Autodesk Inventor part; units mm, degrees
ref_plane "YZ Plane" through (0, 0, 0) normal (1, 0, 0) x (0, 1, 0)
ref_plane "XZ Plane" through (0, 0, 0) normal (0, 1, 0) x (-1, 0, 0)
ref_plane "XY Plane" through (0, 0, 0) normal (0, 0, 1) x (1, 0, 0)
sketch "Sketch1" plane through (0, 0, 0) normal (0, 0, 1) x (1, 0, 0)
  circle A0 centre (0, 0) radius 75
  line L0 (-90.1494, 78.9771) -> (78.0254, 78.9771) construction
  line L1 (78.0254, 78.9771) -> (78.0254, -87.6961) construction
  line L2 (78.0254, -87.6961) -> (-90.1494, -87.6961) construction
  line L3 (-90.1494, -87.6961) -> (-90.1494, 78.9771) construction
  line L4 (-5, 62.2697) -> (-5, 20.6534)
  line L5 (5, 20.6534) -> (5, 59.1608)
  line L6 (15.3864, 14.6568) -> (53.6249, 36.7338)
  line L7 (58.6249, 28.0736) -> (20.3864, 5.9966)
  line L8 (20.3864, -5.9966) -> (58.6249, -28.0736)
  line L9 (15.3864, -14.6568) -> (53.6249, -36.7338)
  line L10 (5, -20.6534) -> (5, -64.8074)
  line L11 (-5, -64.8074) -> (-5, -20.6534)
  line L12 (-15.3864, -14.6568) -> (-53.6249, -36.7338)
  line L13 (-58.6249, -28.0736) -> (-20.3864, -5.9966)
  line L14 (-20.3864, 5.9966) -> (-58.6249, 28.0736)
  line L15 (-53.6249, 36.7338) -> (-15.3864, 14.6568)
  line L16 (5, 59.1608) -> (5, 64.8074)
  line L17 (-5, 62.2697) -> (-5, 64.8074)
  arc A1 (10.8333, 64.0909) -> (5, 59.1608) centre (10, 59.1608) ccw
  arc A2 (-5, 64.8074) -> (-53.6249, 36.7338) centre (0, 0) ccw
  arc A3 (-5, 20.6534) -> (-15.3864, 14.6568) centre (0, 0) ccw
  arc A4 (15.3864, 14.6568) -> (5, 20.6534) centre (0, 0) ccw
  arc A5 (53.6249, 36.7338) -> (5, 64.8074) centre (0, 0) ccw
  arc A6 (58.6249, -28.0736) -> (58.6249, 28.0736) centre (0, 0) ccw
  arc A7 (20.3864, -5.9966) -> (20.3864, 5.9966) centre (0, 0) ccw
  arc A8 (5, -20.6534) -> (15.3864, -14.6568) centre (0, 0) ccw
  arc A9 (5, -64.8074) -> (53.6249, -36.7338) centre (0, 0) ccw
  arc A10 (-20.3864, 5.9966) -> (-20.3864, -5.9966) centre (0, 0) ccw
  arc A11 (-15.3864, -14.6568) -> (-5, -20.6534) centre (0, 0) ccw
  arc A12 (-58.6249, 28.0736) -> (-58.6249, -28.0736) centre (0, 0) ccw
  arc A13 (-53.6249, -36.7338) -> (-5, -64.8074) centre (0, 0) ccw
  line L18 (5, 2.8868) -> (5, -2.8868)
  line L19 (-5, 2.8868) -> (0, 5.7735)
  line L20 (5, 2.8868) -> (0, 5.7735)
  line L21 (-5, 2.8868) -> (-5, -2.8868)
  line L22 (0, -5.7735) -> (5, -2.8868)
  line L23 (-5, -2.8868) -> (0, -5.7735)
  line L24 (0, 0) -> (0, 5.7735)
  dimension "d5" = 150
  dimension "d41" = 10
  dimension "d54" = 5
  dimension "d74" = 120
  dimension "d76" = 120
  dimension "d77" = 120
  dimension "d78" = 120
  dimension "d79" = 120
  dimension "d80" = 120
  dimension "d81" = 10
extrude "Extrusion1" add sketch "Sketch1" along normal blind 6
fillet "Fillet1" radius 5 1 edges at (5, 64.8074, 3)
fillet "Fillet2" radius 5 23 edges at (-53.6249, 36.7338, 3) (5, 20.6534, 3) (-53.6249, -36.7338, 3) (-58.6249, -28.0736, 3) (5, -64.8074, 3) (20.3864, -5.9966, 3) (15.3864, 14.6568, 3) (20.3864, 5.9966, 3) (15.3864, -14.6568, 3) (5, -20.6534, 3) (-20.3864, 5.9966, 3) (-15.3864, -14.6568, 3) (-5, -20.6534, 3) (53.6249, -36.7338, 3) (58.6249, 28.0736, 3) (-5, 64.8074, 3) (-5, 20.6534, 3) (-15.3864, 14.6568, 3) (58.6249, -28.0736, 3) (53.6249, 36.7338, 3) (-5, -64.8074, 3) (-20.3864, -5.9966, 3) (-58.6249, 28.0736, 3)
equation "\"BendRadius\" = Thickness"
equation "\"BendReliefWidth\" = Thickness"
equation "\"BendReliefDepth\" = 0.5 * Thickness"
equation "\"CornerReliefSize\" = 4 * Thickness"
equation "\"MinimumRemnant\" = 2 * Thickness"
equation "\"TransitionRadius\" = BendRadius"
equation "\"JacobiRadiusSize\" = BendRadius"
equation "\"GapSize\" = Thickness"
properties part number "wheel" material "Hardboard"
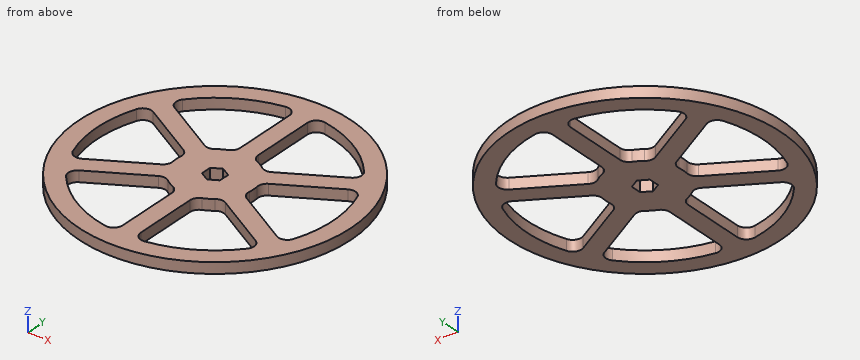
CAD build for the part. Positions are in the model's coordinates, mm. Coordinates: 2 decimals unless noted, no trailing zeros. Order: outer loops, then holes, each group sorted by start corner. A loop starts at its lowest first (then second) coordinate and runs counter-clockwise, first axis right, second up. Notation, with made-up numbers: M 67.5,86 L 99.5,86 A21 cw 99.5,114 Z; hole C 17,67 d10. An arc over 180 degrees is marked long. Write each question's results on one line, items separated by ' | '. Start each with the question number.
Q1. Flat gauge pins, fed straight in: P1, Ø3, axis at y = 37.5, z = 2, coming from the +X side; P2, Ø2, axis at x = -56.5, z = 5, coming from the -Y side; P3, Ø1.5, axis at x = 54.5, z = 3, coming from the -Y side; P4, Ø12, axis at x = -29.5, y = -45, coming from the +Z side. Where does each tip first touch, or does it go through?
Q2. Drill centre lines: probe 1 along X at (y, z) = (-1, 5.75); probe 2 along X at (y, z) = (12, 5); probe 3 along X at (y, z) = (57, 0.75). Where is each one in solid material? Low to high. Write a range as from..to.
Q3. Cut at C-C (y = -57). List the corners of the cut face in (x, z).
Q4. Cut at A-A (y = 0). List the corners of the cut face in (x, z), then the cut area to 3 significant figures.
Q5. Cut at D-D (z = 2.25). Count the separate pieces of the cut face and the enclosed holes in it, then the cut area to 3 significant figures.
Q6. Cut at B-B (x = -16). List the corners of the cut face in (y, z), then the cut area to 3 significant figures.
Found:
1) P1: x = 65.8 | P2: y = -50.45 | P3: y = -52.31 | P4: through
2) probe 1: -74.99..-64.99, -21.23..-5, 5..21.23, 64.99..74.99 | probe 2: -74.03..-63.88, -30.78..30.78, 63.88..74.03 | probe 3: -48.74..-31.24, -5..5, 31.24..48.74
3) outline: M -48.74,0 L -31.24,0 L -31.24,6 L -48.74,6 Z; M -5,0 L 5,0 L 5,6 L -5,6 Z; M 31.24,0 L 48.74,0 L 48.74,6 L 31.24,6 Z
4) outline: M -75,0 L -65,0 L -65,6 L -75,6 Z; M -21.25,0 L -5,0 L -5,6 L -21.25,6 Z; M 5,0 L 21.25,0 L 21.25,6 L 5,6 Z; M 65,0 L 75,0 L 75,6 L 65,6 Z | area: 315 mm²
5) separate pieces: 1 | enclosed holes: 7 | area: 8,480 mm²
6) outline: M -73.27,0 L -63,0 L -63,6 L -73.27,6 Z; M -15.8,0 L 15.8,0 L 15.8,6 L -15.8,6 Z; M 63,0 L 73.27,0 L 73.27,6 L 63,6 Z | area: 313 mm²
